```python
from build123d import *

# Parameters (mm, degrees)
SKIZZE1_R                       = 1.6
AUFSATZ_LINEAR_AUSTRAGEN1_DEPTH = 5
SKIZZE2_R                       = 3
SCHNITT_LINEAR_AUSTRAGEN1_DEPTH = 2.5


with BuildPart() as part:
    # Skizze1 → Aufsatz-Linear austragen1 (new body)
    with BuildSketch(Plane(origin=(0, 0, 0), x_dir=(1, 0, 0), z_dir=(0, 1, 0))):
        with BuildLine():
            Line((-11.407603893, 26.585350281), (11.592396107, 36.585350281))
            ThreePointArc((11.592396107, 36.585350281), (17.315272821, 35.330573989), (17.917777995, 29.502815505))
            Line((17.917777995, 29.502815505), (6.526122928, 14.921747017))
            ThreePointArc((6.526122928, 14.921747017), (6.199926496, 14.320953091), (6.087096426, 13.646692883))
            Line((6.087096426, 13.646692883), (6.087096426, -13.646692883))
            ThreePointArc((6.087096426, -13.646692883), (6.199926496, -14.320953091), (6.526122928, -14.921747017))
            Line((6.526122928, -14.921747017), (17.917777995, -29.502815505))
            ThreePointArc((17.917777995, -29.502815505), (17.315272821, -35.330573989), (11.592396107, -36.585350281))
            Line((11.592396107, -36.585350281), (-11.407603893, -26.585350281))
            ThreePointArc((-11.407603893, -26.585350281), (-13.595369801, -24.741518486), (-14.413973336, -22))
            Line((-14.413973336, -22), (-14.413973336, 22))
            ThreePointArc((-14.413973336, 22), (-13.595369801, 24.741518486), (-11.407603893, 26.585350281))
        make_face()
        with Locations(Location((-9.413973336, 22, 0), (0, 0, 270))):
            Circle(SKIZZE1_R, mode=Mode.SUBTRACT)
        with Locations(Location((13.586026664, 32, 0), (0, 0, 270))):
            Circle(SKIZZE1_R, mode=Mode.SUBTRACT)
        with Locations(Location((2.586026664, 18, 0), (0, 0, 270))):
            Circle(SKIZZE1_R, mode=Mode.SUBTRACT)
        with Locations(Location((2.586026664, -18, 0), (0, 0, 90))):
            Circle(SKIZZE1_R, mode=Mode.SUBTRACT)
        with Locations(Location((13.586026664, -32, 0), (0, 0, 90))):
            Circle(SKIZZE1_R, mode=Mode.SUBTRACT)
        with Locations(Location((-9.413973336, -22, 0), (0, 0, 90))):
            Circle(SKIZZE1_R, mode=Mode.SUBTRACT)
        with BuildLine():
            Line((-9.413973336, 10.935684827), (-9.413973336, -10.935684827))
            ThreePointArc((-9.413973336, -10.935684827), (-4.413973336, -15.935684827), (0.586026664, -10.935684827))
            Line((0.586026664, -10.935684827), (0.586026664, 10.935684827))
            ThreePointArc((0.586026664, 10.935684827), (-4.413973336, 15.935684827), (-9.413973336, 10.935684827))
        make_face(mode=Mode.SUBTRACT)
    extrude(amount=AUFSATZ_LINEAR_AUSTRAGEN1_DEPTH)

    # Skizze2 → Schnitt-Linear austragen1 (cut)
    with BuildSketch(Plane.XZ):
        with Locations(Location((2.586026664, -18, 0), (0, 0, 270))):
            Circle(SKIZZE2_R)
        with Locations(Location((2.586026664, 18, 0), (0, 0, 270))):
            Circle(SKIZZE2_R)
    extrude(amount=-SCHNITT_LINEAR_AUSTRAGEN1_DEPTH, mode=Mode.SUBTRACT)


solid = part.part
```
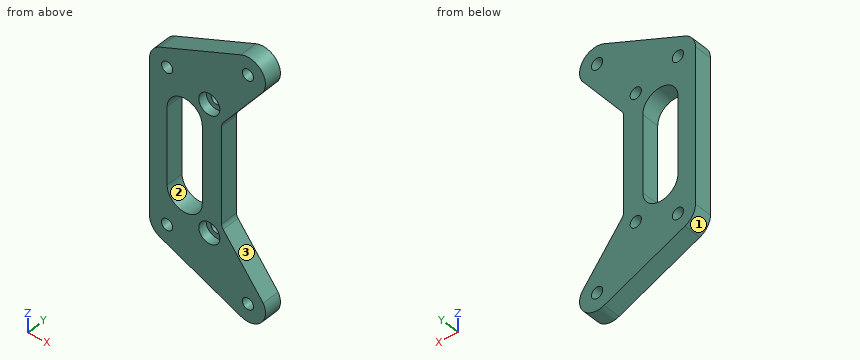
Build history of the part. All positions in model axes, mm. Face numbers are marked on the shaded views. A direction names the side the tool comes from. Round coordinates to 2 decimals unless told otherwise and drop trailing zeros. Loops run counter-clockwise (first coordinate to the right, second up) from the corner with the lowest first, then second, coordinate; pieces in that order, holes last. Notation, with made-up numbers: M -1,30.25 L 20,30.25 A11 ccw 20,39.25 Z; hole C 71,-39.75 d4. An arc over 180 degrees is marked long. Answer as CSV lines item,"result".
1. Flat gauge pins, fed straight in: P1, Ø1.8, axis at x = 3, z = 18, coming from the -Y side; P2, Ø2, axis at y = 3.5, z = -25.5, coming from the -X side; P3, Ø3, axis at x = 8.5, y = 3, coming from the -Z side; P4, Ø2.5, axis at y = 2.5, z = -1.5, coming from the +X side. Where does each tip first touch, or does it go through?
Resolved:
P1,"passes through"
P2,"stops at x = -13.74"
P3,"stops at z = -35.89"
P4,"stops at x = 6.09"
2. Cut at B-B on x = -6.5. Write the cut outline in (y, z), then the cut area to 3 significant figures.
Resolved:
outline,"M 0,-28.72 L 5,-28.72 L 5,-15.48 L 0,-15.48 Z; M 0,15.48 L 5,15.48 L 5,28.72 L 0,28.72 Z"
area,"132 mm²"
3. Cut at A-A on z = 2.5. Write the cut outline in (x, y), then the cut area to 3 significant figures.
Resolved:
outline,"M -14.41,0 L -9.41,0 L -9.41,5 L -14.41,5 Z; M 0.59,0 L 6.09,0 L 6.09,5 L 0.59,5 Z"
area,"52.5 mm²"
4. 3-axis set-ups, long thin cutter, end or side, ignore diameter. For the marked faces 1, 2 and 3: which of +Z, -Z, +X, -X, +Y, -Y reach the whole face in a straight line?
Resolved:
face 1,"-Z, -X, +Y, -Y"
face 2,"+Y, -Y"
face 3,"+X, +Y, -Y"
5. Wall check: probe 1 along X at (y, z) = (3.45, 7.5); probe 2 along Z at (x, y) = (13, 4.4); probe 3 along Z at (x, y) = (-9.5, 4.65). Give the ranges that are in metal, low to high. Write a range as [from, to].
Resolved:
probe 1,"x = [-14.41, -9.41], [0.59, 6.09]"
probe 2,"z = [-36.97, -33.49], [-30.51, -23.21], [23.21, 30.51], [33.49, 36.97]"
probe 3,"z = [-27.41, -23.6], [-20.4, 20.4], [23.6, 27.41]"
6. Cut at D-D on z = 18. Write the cut outline in (x, y), then the cut area to 3 significant figures.
Resolved:
outline,"M -14.41,0 L -0.41,0 L -0.41,2.5 L 0.99,2.5 L 0.99,5 L -14.41,5 Z; M 4.19,2.5 L 5.59,2.5 L 5.59,0 L 8.93,0 L 8.93,5 L 4.19,5 Z"
area,"93.7 mm²"
7. Cut at C-C on y = 0.8. Write the cut outline in (x, z).
Resolved:
outline,"M -14.41,-22 A5 ccw -11.41,-26.59 L 11.59,-36.59 A5 ccw 17.92,-29.5 L 6.53,-14.92 A2.07 cw 6.09,-13.65 L 6.09,13.65 A2.07 cw 6.53,14.92 L 17.92,29.5 A5 ccw 11.59,36.59 L -11.41,26.59 A5 ccw -14.41,22 Z; hole C -9.41,-22 d3.2; hole C -9.41,22 d3.2; hole M -9.41,-10.94 A5 ccw 0.59,-10.94 L 0.59,10.94 A5 ccw -9.41,10.94 Z; hole C 2.59,-18 d6; hole C 2.59,18 d6; hole C 13.59,-32 d3.2; hole C 13.59,32 d3.2"
